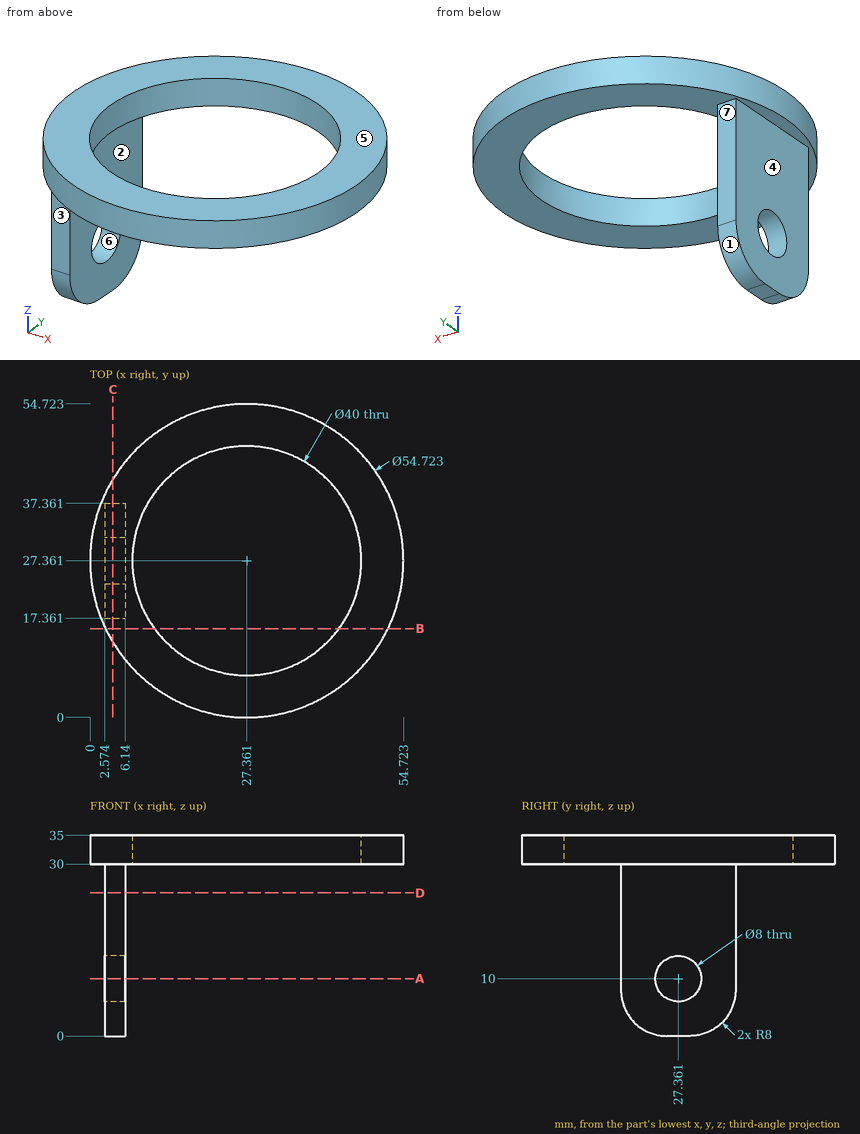
Geometry check sheet. Reference: drawing and pictorial views, mm from the part's lowest x, y, z. A direction names the side the tool comes from. Round coordinates to 2 decimals unless told otherwise and drop trailing zeros. Loops run counter-clockwise (first coordinate to the right, second up) from the corner with the lowest first, then second, coordinate; pieces in that order, holes last. Notation, with made-up numbers: (55.5, 20) -> (110.5, 20) arc R24 cw to (110.5, 36) -> close; hole circle Ø6 at (53, -12). An arc over 180 degrees is marked (long way). Answer as a JSON object with one key per item and string values.
Q1. Section check C-C (x = 4). Record the boundary of the cut face in (y, z) (1 decimal), then the cut area to 3 significant figures.
Data:
{"outline": "(13.1, 30) -> (17.4, 30) -> (17.4, 8) arc R8 ccw to (25.4, 0) -> (29.4, 0) arc R8 ccw to (37.4, 8) -> (37.4, 30) -> (41.6, 30) -> (41.6, 35) -> (13.1, 35) -> close; hole circle Ø8 at (27.4, 10)", "area": "665 mm2"}
Q2. Scan lines: line 1 (Z direction, x = 3, y = 27); line 2 (X direction, y = 33.5, z = 15) (1 decimal); line 3 (Z direction, x = 46.5, y = 12). Record each from-to range of solid material in increasing order. Write a range as from..to.
Data:
{"line 1": "z = 0..6.02, 13.98..35", "line 2": "x = 2.6..6.1", "line 3": "z = 30..35"}
Q3. Draft check along Y on the marked faces 5, 6 and 7. Enter one of: pulls with the +Y half, pulls with the -Y half, needs draft (parallel to the pull), parting line crosses it, or undercut.
Data:
{"face 5": "needs draft", "face 6": "undercut", "face 7": "pulls with the +Y half"}
Q4. Access from +Z, -Z, +X, -X, +Y, -Y to the whole of each face (thin tool, end or side, straight path). Record for the marked faces 1, 2, 3 and 4.
Data:
{"face 1": "-Z, +X, -X, +Y", "face 2": "-Z, +X, +Y, -Y", "face 3": "-Z, +X, -X, -Y", "face 4": "-Z, -X, +Y, -Y"}
Q5. Section check A-A (z = 10). Record the boundary of the cut face in (x, y) (1 decimal), then the cut area to 3 significant figures.
Data:
{"outline": "(2.6, 17.4) -> (6.1, 17.4) -> (6.1, 23.4) -> (2.6, 23.4) -> close; (2.6, 31.4) -> (6.1, 31.4) -> (6.1, 37.4) -> (2.6, 37.4) -> close", "area": "42.8 mm2"}
Q6. Section check D-D (z = 25). Record the boundary of the cut face in (x, y) (1 decimal).
Data:
{"outline": "(2.6, 17.4) -> (6.1, 17.4) -> (6.1, 37.4) -> (2.6, 37.4) -> close"}
Q7. Go/stop test with flat-tipped pins: P1, Ø10, axis at y = 28, z = 22.5, coming from the +X side; P2, Ø8, axis at y = 42.5, z = 3.5, coming from the +X side; P3, Ø5, axis at y = 34, z = 16, coming from the -X side; P4, Ø8, axis at x = 16, y = 40, coming from the -Z side. Record where each tip stops, or that it passes through.
Data:
{"P1": "stops at x = 6.14", "P2": "passes through", "P3": "stops at x = 2.57", "P4": "stops at z = 30"}
Q8. Section check B-B (y = 15.5). Record the boundary of the cut face in (x, z) (1 decimal).
Data:
{"outline": "(2.7, 30) -> (11.3, 30) -> (11.3, 35) -> (2.7, 35) -> close; (43.5, 30) -> (52, 30) -> (52, 35) -> (43.5, 35) -> close"}
